from build123d import *

# Parameters (mm, degrees)
SKETCH_1_R          = 6
EXTRUDE_1_DEPTH     = 23
SKETCH_2_R          = 7
EXTRUDE_2_DEPTH     = 2
SKETCH_3_W          = 0.25
SKETCH_3_H          = 1.1
SKETCH_4_R          = 3
CUT_EXTRUDE_1_DEPTH = 27


with BuildPart() as part:
    # 草图1 → 凸台-拉伸1 (new body)
    with BuildSketch(Plane.XY):
        Circle(SKETCH_1_R)
    extrude(amount=EXTRUDE_1_DEPTH)

    # 草图2 → 凸台-拉伸2 (add)
    with BuildSketch(Plane(origin=(0, 0, 0), x_dir=(-1, 0, 0), z_dir=(0, 0, -1))):
        Circle(SKETCH_2_R)
    extrude(amount=EXTRUDE_2_DEPTH)

    # 草图3 → 切除-旋转1 (revolve, cut)
    with BuildSketch(Plane(origin=(0, 0, 0), x_dir=(1, 0, 0), z_dir=(0, 1, 0)), mode=Mode.PRIVATE) as cut_revolve_1_sk:
        with Locations((-5.875, -20.55)):
            Rectangle(SKETCH_3_W, SKETCH_3_H)
    revolve(cut_revolve_1_sk.sketch.rotate(Axis((0, 0, 23), (0, 0, -1)), 180), axis=Axis((0, 0, 23), (0, 0, -1)), mode=Mode.SUBTRACT)

    # 草图4 → 切除-拉伸1 (cut)
    with BuildSketch(Plane(origin=(0, 0, -2), x_dir=(-1, 0, 0), z_dir=(0, 0, -1))):
        Circle(SKETCH_4_R)
    extrude(amount=-CUT_EXTRUDE_1_DEPTH, mode=Mode.SUBTRACT)


solid = part.part
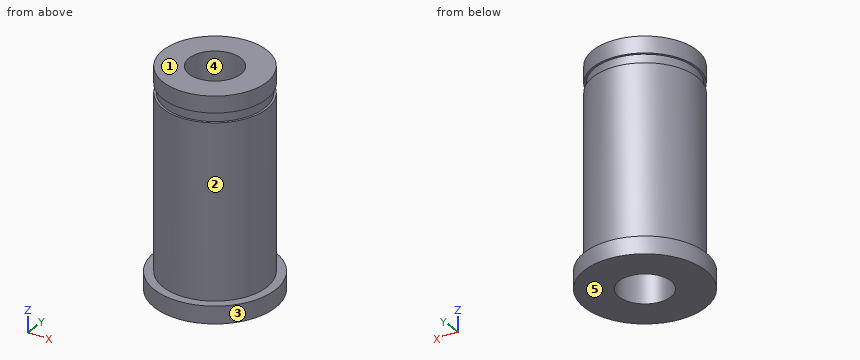
Model file for the job. Use its own axes, mm. Face numbers are marked on the shaded views. A direction names the side the tool comes from. Round coordinates to 2 decimals unless told otherwise and drop trailing zeros. Loops run counter-clockwise (first coordinate to the right, second up) from the corner with the lowest first, then second, coordinate; pieces in that order, holes last. Notation, with made-up numbers: M -3,-11.75 L 2,-11.75 A15 ccw 2,-0.75 Z; hole C -23,56.25 d5. An arc over 180 degrees is marked long. One line per question, with ' | ' between items.
1) Flat gauge pins, fed straight in: pin 1 (4 mm diameter, centred on x = -1, z = 19, fed in from -Y); pin 2 (5 mm diameter, centred on x = 0, y = 0, fed in from +Z); pin 3 (6 mm diameter, centred on x = 4, z = 7, fed in from +Y); pin 4 (1.5 mm diameter, centred on x = 2.5, z = 8.5, fed in from +Y). Where does each tip first touch, or does it go through?
Solved:
pin 1: stops at y = -6 | pin 2: passes through | pin 3: stops at y = 5.92 | pin 4: stops at y = 5.74
2) Drill centre lines: line 1 along Y through (x, z) = (0, 12.5); line 2 along X through (y, z) = (-1.75, 20.75); line 3 along X through (y, z) = (1, 14.25). Where is each one in solid material? Low to high.
Solved:
line 1: y = -6 to -3, 3 to 6 | line 2: x = -5.48 to -2.44, 2.44 to 5.48 | line 3: x = -5.92 to -2.83, 2.83 to 5.92
3) Band-saw the part on A-A (y = 0). Give the cut face in (x, z).
Solved:
outline: M -7,-2 L -3,-2 L -3,23 L -6,23 L -6,21.1 L -5.75,21.1 L -5.75,20 L -6,20 L -6,0 L -7,0 Z; M 3,-2 L 7,-2 L 7,0 L 6,0 L 6,20 L 5.75,20 L 5.75,21.1 L 6,21.1 L 6,23 L 3,23 Z
4) 3-axis set-ups, long thin cutter, end or side, ignore diameter. For the marked faces 1 and 2: which of +Z, -Z, +X, -X, +Y, -Y reach the whole face in a straight line?
Solved:
face 1: +Z, +X, -X, +Y, -Y | face 2: +Z
5) Mould opens along X. For the marked faces 3, 4 and 5 say: +X half, -X half, draft (parallel to the pull), parting line (faces both ways), or undercut.
Solved:
face 3: parting line | face 4: undercut | face 5: draft
6) Band-saw the part on D-D (y = 5.25). Give the cut face in (x, z).
Solved:
outline: M -4.63,-2 L 4.63,-2 L 4.63,0 L 2.9,0 L 2.9,20 L 2.35,20 L 2.35,21.1 L 2.9,21.1 L 2.9,23 L -2.9,23 L -2.9,21.1 L -2.35,21.1 L -2.35,20 L -2.9,20 L -2.9,0 L -4.63,0 Z
7) Band-saw the part on C-C (z = 14). Give the cut face in (x, y), then the cut area to 3 significant figures.
Solved:
outline: C 0,0 d12; hole C 0,0 d6 | area: 84.8 mm²
